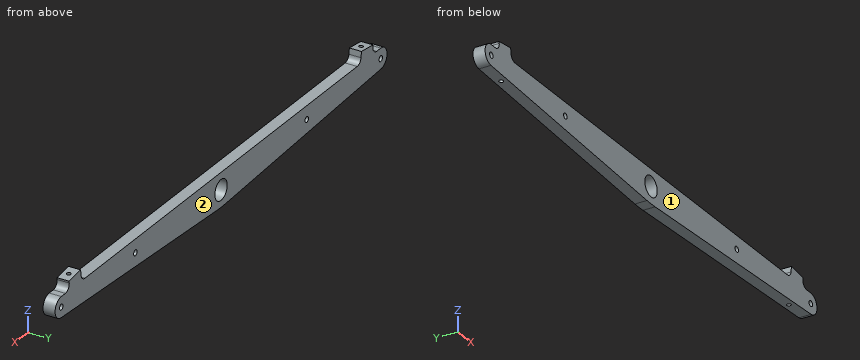
from build123d import *

# Parameters (mm, degrees)
STOCK_UOR22_CNS_5_P_007_SWING_ARM_PLATE_START = -3.175
STOCK_UOR22_CNS_5_P_007_SWING_ARM_PL_2_R      = 2.9
STOCK_UOR22_CNS_5_P_007_SWING_ARM_PL_2_R_2    = 2.25
STOCK_UOR22_CNS_5_P_007_SWING_ARM_PL_2_R_3    = 8
STOCK_UOR22_CNS_5_P_007_SWING_ARM_PLATE_DEPTH = 3.175
BOSS_EXTRUDE2_DEPTH                           = 9.525
SKETCH5_R                                     = 8
CUT_EXTRUDE1_DEPTH                            = 235.085039959
SKETCH7_R                                     = 2.25
CUT_EXTRUDE3_DEPTH                            = 235.085039959
CUT_EXTRUDE2_DEPTH                            = 235.085039959
BOSS_EXTRUDE5_DEPTH                           = 9.525
M4_TAPPED_HOLE1_D                             = 3.3
FILLET4_R                                     = 5
FILLET4_OF_MIRROR7_R                          = 5


# Read off the part's stored shape, not the designer's step: Stock-UOR22-CNS-5-P-007_Swing_arm_plate-1
with BuildPart() as part:
    # Stock-UOR22-CNS-5-P-007_Swing_arm_pl 2 → Stock-UOR22-CNS-5-P-007_Swing_arm_plate-1 (new body)
    with BuildSketch(Plane(origin=(0, 0, 0), x_dir=(1, 0, 0), z_dir=(0, 1, 0)).offset(STOCK_UOR22_CNS_5_P_007_SWING_ARM_PLATE_START)):
        with BuildLine():
            ThreePointArc((226, -13.432371654), (233.502570944, -6.12369062), (226.392788824, 1.567628346))
            Line((226.392788824, 1.567628346), (5.233595624, 13.15809053))
            ThreePointArc((5.233595624, 13.15809053), (0, 13.295137054), (-5.233595624, 13.15809053))
            Line((-5.233595624, 13.15809053), (-226.392788824, 1.567628346))
            ThreePointArc((-226.392788824, 1.567628346), (-233.502570944, -6.12369062), (-226, -13.432371654))
            Line((-226, -13.432371654), (226, -13.432371654))
        make_face()
        with Locations((-226, -5.927228885)):
            Circle(STOCK_UOR22_CNS_5_P_007_SWING_ARM_PL_2_R, mode=Mode.SUBTRACT)
        with Locations((-206, -5.40297223)):
            Circle(STOCK_UOR22_CNS_5_P_007_SWING_ARM_PL_2_R_2, mode=Mode.SUBTRACT)
        with BuildLine():
            ThreePointArc((-200.009372106, -5.067744788), (-199.5011525, -3.620374273), (-198.117168054, -2.958743238))
            Line((-198.117168054, -2.958743238), (-118.332872644, 1.222574507))
            ThreePointArc((-118.332872644, 1.222574507), (-116.669449692, 0.478429636), (-116.300073603, -1.306027932))
            ThreePointArc((-116.300073603, -1.306027932), (-116.513571396, -3.059574073), (-116.207168794, -4.799293251))
            ThreePointArc((-116.207168794, -4.799293251), (-116.481651343, -6.601525877), (-118.104327652, -7.432371654))
            Line((-118.104327652, -7.432371654), (-198.000054021, -7.432371654))
            ThreePointArc((-198.000054021, -7.432371654), (-199.416863766, -6.843984258), (-200.000040515, -5.425021798))
            ThreePointArc((-200.000040515, -5.425021798), (-200.002045504, -5.246313796), (-200.009372106, -5.067744788))
        make_face(mode=Mode.SUBTRACT)
        with Locations((-110.515692218, -2.900058041)):
            Circle(STOCK_UOR22_CNS_5_P_007_SWING_ARM_PL_2_R_2, mode=Mode.SUBTRACT)
        with BuildLine():
            ThreePointArc((-15.423577727, 6.615822121), (-13.745275303, 5.852940228), (-13.404042587, 4.04124267))
            ThreePointArc((-13.404042587, 4.04124267), (-13.994975846, -0.375034774), (-13.168367384, -4.753325197))
            ThreePointArc((-13.168367384, -4.753325197), (-13.412783431, -6.581699085), (-15.049562725, -7.432371654))
            Line((-15.049562725, -7.432371654), (-102.927056783, -7.432371654))
            ThreePointArc((-102.927056783, -7.432371654), (-104.549733092, -6.601525877), (-104.824215641, -4.799293251))
            ThreePointArc((-104.824215641, -4.799293251), (-104.5176845, -2.745450719), (-104.929619796, -0.710127699))
            ThreePointArc((-104.929619796, -0.710127699), (-104.748793796, 1.103164739), (-103.172267568, 2.017108151))
            Line((-103.172267568, 2.017108151), (-15.423577727, 6.615822121))
        make_face(mode=Mode.SUBTRACT)
        with Locations((110.515692218, -2.900058041)):
            Circle(STOCK_UOR22_CNS_5_P_007_SWING_ARM_PL_2_R_2, mode=Mode.SUBTRACT)
        with BuildLine():
            Line((15.423577727, 6.615822121), (103.172267568, 2.017108151))
            ThreePointArc((103.172267568, 2.017108151), (104.748793796, 1.103164739), (104.929619796, -0.710127699))
            ThreePointArc((104.929619796, -0.710127699), (104.5176845, -2.745450719), (104.824215641, -4.799293251))
            ThreePointArc((104.824215641, -4.799293251), (104.549733092, -6.601525877), (102.927056783, -7.432371654))
            Line((102.927056783, -7.432371654), (15.049562725, -7.432371654))
            ThreePointArc((15.049562725, -7.432371654), (13.412783431, -6.581699085), (13.168367384, -4.753325197))
            ThreePointArc((13.168367384, -4.753325197), (13.994975846, -0.375034774), (13.404042587, 4.04124267))
            ThreePointArc((13.404042587, 4.04124267), (13.745275303, 5.852940228), (15.423577727, 6.615822121))
        make_face(mode=Mode.SUBTRACT)
        with Locations((226, -5.927228885)):
            Circle(STOCK_UOR22_CNS_5_P_007_SWING_ARM_PL_2_R, mode=Mode.SUBTRACT)
        with Locations((206, -5.40297223)):
            Circle(STOCK_UOR22_CNS_5_P_007_SWING_ARM_PL_2_R_2, mode=Mode.SUBTRACT)
        with BuildLine():
            Line((118.332872644, 1.222574507), (198.117168054, -2.958743238))
            ThreePointArc((198.117168054, -2.958743238), (199.5011525, -3.620374273), (200.009372106, -5.067744788))
            ThreePointArc((200.009372106, -5.067744788), (200.002045504, -5.246313796), (200.000040515, -5.425021798))
            ThreePointArc((200.000040515, -5.425021798), (199.416863766, -6.843984258), (198.000054021, -7.432371654))
            Line((198.000054021, -7.432371654), (118.104327652, -7.432371654))
            ThreePointArc((118.104327652, -7.432371654), (116.481651343, -6.601525877), (116.207168794, -4.799293251))
            ThreePointArc((116.207168794, -4.799293251), (116.513571396, -3.059574073), (116.300073603, -1.306027932))
            ThreePointArc((116.300073603, -1.306027932), (116.669449692, 0.478429636), (118.332872644, 1.222574507))
        make_face(mode=Mode.SUBTRACT)
        Circle(STOCK_UOR22_CNS_5_P_007_SWING_ARM_PL_2_R_3, mode=Mode.SUBTRACT)
    extrude(amount=STOCK_UOR22_CNS_5_P_007_SWING_ARM_PLATE_DEPTH)


with BuildPart() as body_2:
    # Sketch3 → Boss-Extrude2 (new body)
    with BuildSketch(Plane(origin=(0, 0, 0), x_dir=(1, 0, 0), z_dir=(0, 1, 0))):
        with BuildLine():
            Line((226.392788824, 1.567628346), (5.233595624, 13.15809053))
            ThreePointArc((5.233595624, 13.15809053), (0, 13.295137054), (-5.233595624, 13.15809053))
            Line((-5.233595624, 13.15809053), (-226.392788824, 1.567628346))
            ThreePointArc((-226.392788824, 1.567628346), (-233.502570944, -6.12369062), (-226, -13.432371654))
            Line((-226, -13.432371654), (226, -13.432371654))
            ThreePointArc((226, -13.432371654), (233.502570944, -6.12369062), (226.392788824, 1.567628346))
        make_face()
    extrude(amount=BOSS_EXTRUDE2_DEPTH)

    # Sketch5 → Cut-Extrude1 (cut, through all)
    with BuildSketch(Plane.XZ):
        with Locations(Location((0, 0, 0), (0, 0, 270))):
            Circle(SKETCH5_R)
    extrude(amount=-CUT_EXTRUDE1_DEPTH, mode=Mode.SUBTRACT)

    # Sketch7 → Cut-Extrude3 (cut, through all)
    with BuildSketch(Plane.XZ):
        with Locations(Location((-206, 5.40297223, 0), (0, 0, 270))):
            Circle(SKETCH7_R)
        with Locations(Location((-110.515692218, 2.900058041, 0), (0, 0, 270))):
            Circle(SKETCH7_R)
    cut_extrude3 = extrude(amount=-CUT_EXTRUDE3_DEPTH, mode=Mode.SUBTRACT)

    # Sketch6 → Cut-Extrude2 (cut, through all)
    with BuildSketch(Plane.XZ):
        with BuildLine():
            Line((-226.392788824, -1.567628346), (-206.420198128, -2.614347471))
            ThreePointArc((-206.420198128, -2.614347471), (-214.02610991, 5.613681539), (-206, 13.432371654))
            Line((-206, 13.432371654), (-226, 13.432371654))
            ThreePointArc((-226, 13.432371654), (-233.502570944, 6.12369062), (-226.392788824, -1.567628346))
        make_face()
    cut_extrude2 = extrude(amount=-CUT_EXTRUDE2_DEPTH, mode=Mode.SUBTRACT)

    # Mirror4: Cut-Extrude3, Cut-Extrude2 across plane
    add(cut_extrude3.mirror(Plane(origin=(0, 0, 0), x_dir=(0, 0, 1), z_dir=(1, 0, 0))), mode=Mode.SUBTRACT)
    add(cut_extrude2.mirror(Plane(origin=(0, 0, 0), x_dir=(0, 0, 1), z_dir=(1, 0, 0))), mode=Mode.SUBTRACT)

    # Sketch8 → Boss-Extrude5 (add)
    with BuildSketch(Plane(origin=(0, 9.525, 0), x_dir=(1, 0, 0), z_dir=(0, 1, 0))):
        Polygon((-180, -13.432371654), (-195.112647382, -13.432371654), (-195.982696315, -20.518351578), (-181.094504041, -22.34639173), align=None)
    boss_extrude5 = extrude(amount=-BOSS_EXTRUDE5_DEPTH)

    # M4 Tapped Hole1 (through all)
    with Locations(Plane(origin=(-5.392681082, 0, 43.919862911), x_dir=(0.992546151641322, 0, 0.12186934340514761), z_dir=(-0.12186934340514761, 0, 0.992546151641322))):
        with Locations((-184.521312982, 4.7625)):
            m4_tapped_hole1 = Hole(M4_TAPPED_HOLE1_D / 2)

    # Fillet4
    fillet4_edges = [body_2.edges().sort_by_distance(p)[0] for p in [
        (-195.112647382, 4.7625, 13.432371654),
        (-180, 4.7625, 13.432371654),
    ]]
    fillet(fillet4_edges, radius=FILLET4_R)

    # Mirror7: Boss-Extrude5, M4 Tapped Hole1 across plane
    add(boss_extrude5.mirror(Plane(origin=(0, 0, 0), x_dir=(0, 0, 1), z_dir=(1, 0, 0))))
    add(m4_tapped_hole1.mirror(Plane(origin=(0, 0, 0), x_dir=(0, 0, 1), z_dir=(1, 0, 0))), mode=Mode.SUBTRACT)

    # Fillet4 of Mirror7
    fillet4_of_mirror7_edges = [body_2.edges().sort_by_distance(p)[0] for p in [
        (195.112647382, 4.7625, 13.432371654),
        (180, 4.7625, 13.432371654),
    ]]
    fillet(fillet4_of_mirror7_edges, radius=FILLET4_OF_MIRROR7_R)


solid = body_2.part
CAD build for the part. Positions are in the model's coordinates, mm. Face numbers are marked on the shaded views. Coordinates: 2 decimals unless noted, no trailing zeros. Write each loop counter-clockwise with the first axis right and the second up, starting at its lowest first coordinate (ties: lowest second). Pieces come first, ordered by that corner, then holes. Notation, with made-up numbers: M -7,64.25 L 9,64.25 A19 ccw 9,101.25 Z; hole C 36.5,-7.5 d4. An arc over 180 degrees is marked long. Return JSON: item names as keys, results as strings.
Item 1: Two-plate mould, pull along Y, no slides. Class the marked faces 1 and 2: +Y half, -Y half, draft (parallel to the pull), parting line (faces both ways), or undercut.
Findings below:
{"face 1": "-Y half", "face 2": "+Y half"}
Item 2: Slice it at A-A, the plane x = 0. Write the cut outline in (y, z) (3 decimals), and give its area (3 significant figures).
Findings below:
{"outline": "M 0,-13.295 L 9.525,-13.295 L 9.525,-8 L 0,-8 Z; M 0,8 L 9.525,8 L 9.525,13.432 L 0,13.432 Z", "area": "102 mm2"}
Item 3: Slice it at B-B, the plane x = -167.5. Write the cut outline in (y, z) (3 decimals).
Findings below:
{"outline": "M 0,-4.654 L 9.525,-4.654 L 9.525,13.432 L 0,13.432 Z"}
Item 4: Slice it at C-C, the plane x = -63. Write the cut outline in (y, z) (3 decimals), and give its area (3 significant figures).
Findings below:
{"outline": "M 0,-10.131 L 9.525,-10.131 L 9.525,13.432 L 0,13.432 Z", "area": "224 mm2"}
Item 5: Drop flat-ended pins along their axis: pin 1 Ø5 at (x, y) = (152.5, 1.5) entering from -Z; pin 2 Ø4 at (x, y) = (202.5, 5.5) entering from +Z; pin 3 Ø1 at (y, z) = (3.5, 8.5) entering from -X. Give the stop position or say it passes through.
Findings below:
{"pin 1": "stops at z = -5.57", "pin 2": "stops at z = 13.44", "pin 3": "stops at x = -213.6"}
Item 6: Probe line 1 (X direction, y = 2, z = 18.5); line 2 (X direction, y = 4.25, z = 3); line 3 (X direction, y = 6.5, z = 2.5). List the from-to ranges inside material, lowest first. Write a range as from..to.
Findings below:
{"line 1": "x = -195.76..-180.62, 180.62..195.76", "line 2": "x = -213.66..-187.86, -184.7..-112.76, -108.27..-7.42, 7.42..108.27, 112.76..184.7, 187.86..213.66", "line 3": "x = -213.49..-112.73, -108.3..-7.6, 7.6..108.3, 112.73..213.49"}
